from build123d import *

# Parameters (mm, degrees)
SKETCH1_R           = 1.65
SKETCH1_R_2         = 7.5
SKETCH1_R_3         = 1
SKETCH1_W           = 4
SKETCH1_H           = 3
SKETCH1_W_2         = 10
SKETCH1_H_2         = 18.5
BOSS_EXTRUDE3_DEPTH = 2.7


with BuildPart() as part:
    # Sketch1 → Boss-Extrude3 (new body)
    with BuildSketch(Plane.XY):
        Polygon((-46.02, -28), (-46.02, -25.3), (-15.34, -25.3), (-15.34, -28), (15.34, -28), (15.34, -25.3), (46.02, -25.3), (46.02, -28), (76.7, -28), (76.7, 99), (-76.7, 99), (-76.7, -28), align=None)
        with Locations((-18.5, 2)):
            Circle(SKETCH1_R, mode=Mode.SUBTRACT)
        with Locations((18.567940233, 2)):
            Circle(SKETCH1_R, mode=Mode.SUBTRACT)
        with Locations((-51.7, 22)):
            Circle(SKETCH1_R_2, mode=Mode.SUBTRACT)
        with Locations((51.7, 22)):
            Circle(SKETCH1_R_2, mode=Mode.SUBTRACT)
        with Locations((10.5, 94.5)):
            Circle(SKETCH1_R_3, mode=Mode.SUBTRACT)
        with Locations((-10.5, 82)):
            Circle(SKETCH1_R_3, mode=Mode.SUBTRACT)
        with Locations((-10.5, 94.5)):
            Circle(SKETCH1_R_3, mode=Mode.SUBTRACT)
        with Locations((10.5, 82)):
            Circle(SKETCH1_R_3, mode=Mode.SUBTRACT)
        with Locations((0, -16)):
            Rectangle(SKETCH1_W, SKETCH1_H, mode=Mode.SUBTRACT)
        with Locations((0, 87.25)):
            Rectangle(SKETCH1_W_2, SKETCH1_H_2, mode=Mode.SUBTRACT)
    extrude(amount=BOSS_EXTRUDE3_DEPTH)


solid = part.part
Can you work these out from the model? Positions are in its coordinate system, mm. Coordinates: 2 decimals unless noted, no trailing zeros. Order: outer loops, then holes, each group sorted by start corner. A loop starts at its lowest first (then second) coordinate and runs counter-clockwise, first axis right, second up. Notation, with made-up numbers: (55, 19.25) -> (112, 19.25) arc R19 ccw to (112, 24.25) -> close; hole circle Ø8 at (-24.75, 89.25). An arc over 180 degrees is marked (long way). Use one line per item in the form item = value.
Q1. Imagine slicing it at B-B, the plane x = -18.5. List the corners of the cut face in (y, z) for me, then the cut area to 3 significant figures.
From the geometry:
outline = (-25.3, 0) -> (0.35, 0) -> (0.35, 2.7) -> (-25.3, 2.7) -> close; (3.65, 0) -> (99, 0) -> (99, 2.7) -> (3.65, 2.7) -> close
area = 327 mm²
Q2. Imagine slicing it at C-C, the plane z = 1.15. Give the number of separate pieces and of enclosed holes in the cut face, then the cut area to 3 significant figures.
From the geometry:
separate_pieces = 1
enclosed_holes = 10
area = 18,700 mm²
Q3. I need wall thicknesses on L1, parallel to Y at x = -10.5, z = 0.75; L2, parallel to X at y = 82, z = 0.75; L3, parallel to Y at x = -51.7, z = 1.5. Which ranges of each line are inside material? Lowest first, please.
From the geometry:
L1 = -28 to 81, 83 to 93.5, 95.5 to 99
L2 = -76.7 to -11.5, -9.5 to -5, 5 to 9.5, 11.5 to 76.7
L3 = -28 to 14.5, 29.5 to 99
Q4. Imagine slicing it at D-D, the plane x = 51.7. List the corners of the cut face in (y, z) for me, then the cut area to 3 significant figures.
From the geometry:
outline = (-28, 0) -> (14.5, 0) -> (14.5, 2.7) -> (-28, 2.7) -> close; (29.5, 0) -> (99, 0) -> (99, 2.7) -> (29.5, 2.7) -> close
area = 302 mm²
Q5. Imagine slicing it at A-A, the plane y = 22. List the corners of the cut face in (x, z) for me.
From the geometry:
outline = (-76.7, 0) -> (-59.2, 0) -> (-59.2, 2.7) -> (-76.7, 2.7) -> close; (-44.2, 0) -> (44.2, 0) -> (44.2, 2.7) -> (-44.2, 2.7) -> close; (59.2, 0) -> (76.7, 0) -> (76.7, 2.7) -> (59.2, 2.7) -> close
